```python
from build123d import *

# Parameters (mm, degrees)
F0_R     = 19.05
F1_DEPTH = 44.45
F0_R_2   = 31.75
F2_DEPTH = 25.4
F3_DEPTH = 25.4


with BuildPart() as f1:
    # F0 (on Front) → F1 (new body)
    with BuildSketch(Plane.XZ):
        Circle(F0_R)
    extrude(amount=F1_DEPTH)

    # F0 (on Front) → F2 (join)
    with BuildSketch(Plane.XZ):
        Circle(F0_R_2)
        Circle(F0_R, mode=Mode.SUBTRACT)
    extrude(amount=F2_DEPTH)

    # F3 (add): a face of the model
    f3_faces = [f1.faces().sort_by_distance(p)[0] for p in [
        (0, -44.45, 0),
    ]]
    extrude(f3_faces, amount=F3_DEPTH)


solid = f1.part
```
Can you work these out from the model? Positions are in its coordinate system, mm. A direction names the side the tool comes from. Round coordinates to 2 decimals unless told otherwise and drop trailing zeros. Loops run counter-clockwise (first coordinate to the right, second up) from the corner with the lowest first, then second, coordinate; pieces in that order, holes last.
Item 1: Suppose I cut it at A-A, the plane z = 0. Write out the boundary of the cut face in (x, y).
Item 2: Will these pins go through, and if not, where does the flat tip stop? pin 1 Ø1.5 at (y, z) = (-49.5, -8) entering from +X; pin 2 Ø6 at (x, z) = (-23.5, -1.5) entering from -Y; pin 3 Ø10 at (y, z) = (-62, 14) entering from +X.
Item 3: Suppose I cut it at C-C, the plane y = -44.5. Write out the boundary of the cut face in (x, z), then the cut area to 3 significant figures.
Item 4: Suppose I cut it at B-B, the plane x = 0. Write out the boundary of the cut face in (y, z), then the cut area to 3 significant figures.
Item 5: Suppose I cut it at D-D, the plane y = -15. Write out the boundary of the cut face in (x, z), then the cut area to 3 significant figures.
Item 6: Please list where these lines run through material, in increasing order: L1, parallel to Y at x = -27, z = 11; L2, parallel to X at y = -23.5, z = 1; L3, parallel to X at y = -49, z = 0.5.
Item 7: Which directions (+Z, -Z, +X, -X, +Y, -Y) give clear straight access to the entire face, cutting with the end or side of a thin tool? Please do faces 1 (the cylindrical face through (-15.12, -47.31, -11.59)), 2 (the flat face through (0, -69.85, 0)).
Reported:
1. outline: (-31.75, -25.4) - (-19.05, -25.4) - (-19.05, -69.85) - (19.05, -69.85) - (19.05, -25.4) - (31.75, -25.4) - (31.75, 0) - (-31.75, 0) - close
2. pin 1: stops at x = 17.62
2. pin 2: stops at y = -25.4
2. pin 3: stops at x = 16.79
3. outline: circle Ø38.1 at (0, 0)
3. area: 1,140 mm2
4. outline: (-69.85, -19.05) - (-25.4, -19.05) - (-25.4, -31.75) - (0, -31.75) - (0, 31.75) - (-25.4, 31.75) - (-25.4, 19.05) - (-69.85, 19.05) - close
4. area: 3,310 mm2
5. outline: circle Ø63.5 at (0, 0)
5. area: 3,170 mm2
6. L1: y = -25.4 to 0
6. L2: x = -31.73 to 31.73
6. L3: x = -19.04 to 19.04
7. face 1: -Y
7. face 2: +Z, -Z, +X, -X, -Y
